For this review, take the finished solid that the model builds, in its own axes (mm). Face numbers are marked on the shaded views. A direction names the side the tool comes from. Give positions to 0.01 mm unless a question says otherwise; leave off trailing zeros. Write each loop counter-clockwise with the first axis right and the second up, starting at its lowest first coordinate (ties: lowest second). Pieces come first, ordered by that corner, then holes. Notation, with made-up numbers: (-37.75, -24.5) -> (2.25, -24.5) arc R14 cw to (2.25, 1.5) -> close; hole circle Ø6 at (21, -39). An arc over 180 degrees is marked (long way). Write item = value, one per line.
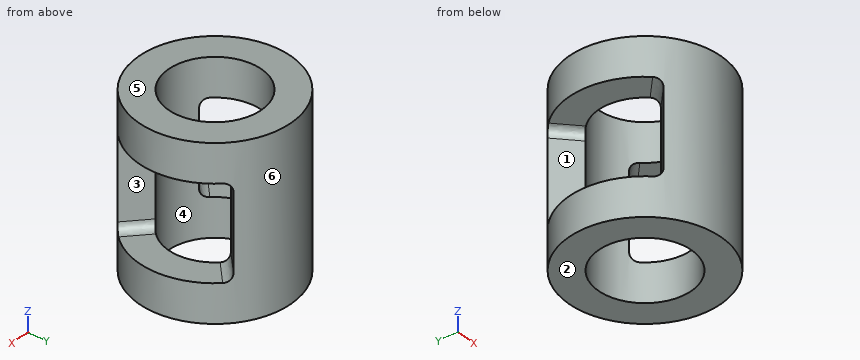
```python
from build123d import *

# Parameters (mm, degrees)
F0_R     = 9
F0_R_2   = 5.5
F1_DEPTH = 20
F2_W     = 3
F2_H     = 11
F4_W     = 40
F4_H     = 11
F6_W     = 40
F6_H     = 11
F9_R     = 1


with BuildPart() as f1:
    # F0 (on Top) → F1 (new body)
    with BuildSketch(Plane.XY):
        Circle(F0_R)
        Circle(F0_R_2, mode=Mode.SUBTRACT)
    extrude(amount=F1_DEPTH)

    # F2 (on Right) → F7 section 0
    with BuildSketch(Plane.YZ):
        with Locations((0, 10)):
            Rectangle(F2_W, F2_H)
    # F4 (on offset) → F7 section 1
    with BuildSketch(Plane.YZ.offset(20)):
        with Locations((0, 10)):
            Rectangle(F4_W, F4_H)
    loft(mode=Mode.SUBTRACT)

    # F2 (on Right) → F8 section 0
    with BuildSketch(Plane.YZ):
        with Locations((0, 10)):
            Rectangle(F2_W, F2_H)
    # F6 (on offset) → F8 section 1
    with BuildSketch(Plane.YZ.offset(-20)):
        with Locations((0, 10)):
            Rectangle(F6_W, F6_H)
    loft(mode=Mode.SUBTRACT)

    # F9
    f9_edges = [f1.edges().sort_by_distance(p)[0] for p in [
        (4.508802, -5.670642, 15.5),
        (4.508802, 5.670642, 15.5),
        (4.508802, 5.670642, 4.5),
        (4.508802, -5.670642, 4.5),
        (-4.508802, 5.670642, 4.5),
        (-4.508802, -5.670642, 4.5),
        (-4.508802, -5.670642, 15.5),
        (-4.508802, 5.670642, 15.5),
    ]]
    fillet(f9_edges, radius=F9_R)


solid = f1.part
```
(1) Tool access review of the marked faces 1, 2 and 3: name each direction out of +Z, -Z, +X, -X, +Y, -Y from which nothing blocks a thin tool from reaching the whole face with its end or side.
Answers below:
face_1 = -X
face_2 = -Z, +X, -X, +Y, -Y
face_3 = +X
(2) Take a section at C-C (z = 2.25). Write out the cut boundary in (x, y).
Answers below:
outline = circle Ø18 at (0, 0); hole circle Ø11 at (0, 0)
(3) To check wall thickness, follow probe 1 along X at (y, z) = (0, 15.75); probe 2 along Z at (x, y) = (-5.75, 1). State the ranges of each line that lie inside material, in increasing order.
Answers below:
probe_1 = -9 to -5.5, 5.5 to 9
probe_2 = 0 to 4.5, 15.5 to 20
(4) Take a section at B-B (x = 0). Write out the cut boundary in (y, z), plus the area to 3 significant figures.
Answers below:
outline = (-9, 0) -> (-5.5, 0) -> (-5.5, 20) -> (-9, 20) -> close; (5.5, 0) -> (9, 0) -> (9, 20) -> (5.5, 20) -> close
area = 140 mm^2
(5) Take a section at A-A (z = 12.25). Write out the cut boundary in (x, y), plus the area to 3 significant figures.
Answers below:
outline = (-5.81, -6.87) arc R9 ccw to (5.81, -6.87) -> (3.21, -4.47) arc R5.5 cw to (-3.21, -4.47) -> close; (-5.81, 6.87) -> (-3.21, 4.47) arc R5.5 cw to (3.21, 4.47) -> (5.81, 6.87) arc R9 ccw to start
area = 68.2 mm^2
(6) Take a section at D-D (y = 0). Count the separate pieces of the cut face and the enclosed holes in it, plus the area to 3 significant figures.
Answers below:
separate_pieces = 4
enclosed_holes = 0
area = 63.0 mm^2
(7) For pin 1 (6 mm diameter, centred on y = 4.5, z = 13.5, fed in from -X); pin 2 (4 mm diameter, centred on y = -3.5, z = 7, fed in from +X); pin 3 (2 mm diameter, centred on y = -4.5, z = 12.5, fed in from -X), all flat-tipped, find the tip position at first contact; note any pin that passes through.
Answers below:
pin_1 = -8.71
pin_2 = 4.32
pin_3 = -4.32
(8) The part is to be moulded in two halves that separate along Y. For the marked faces 4, 5 and 6, say which applies: released by +Y, released by -Y, zero draft, split by the parting line, or undercut.
Answers below:
face_4 = undercut
face_5 = zero draft
face_6 = split by the parting line
